Read the model definition and answer for the solid it produces. Units are mm, in the model's axes. Give positions to 0.01 mm unless a question says otherwise; leave off trailing zeros. Loops run counter-clockwise (first coordinate to the right, second up) from the corner with the lowest first, then second, coordinate; pieces in that order, holes last. Notation, with made-up numbers: (43.5, -13) - (54.5, -13) arc R34 cw to (54.5, 21) - close; hole circle Ø6 at (73, 47). An arc over 180 degrees is marked (long way). Write item = value, one per line.
```python
from build123d import *

# Parameters (mm, degrees)
EXTRUDE_1_DEPTH = 55
FILLET_1_R      = 5


with BuildPart() as part:
    # ｽｹｯﾁ1 → ﾎﾞｽ - 押し出し1 (new body)
    with BuildSketch(Plane.XY):
        with BuildLine():
            Line((61.949000384, 214.222597667), (62.393477517, 215.75962079))
            ThreePointArc((62.393477517, 215.75962079), (0, 224.6), (-62.393477517, 215.75962079))
            Line((-62.393477517, 215.75962079), (-61.949000384, 214.222597667))
            ThreePointArc((-61.949000384, 214.222597667), (0, 223), (61.949000384, 214.222597667))
        make_face()
    extrude(amount=EXTRUDE_1_DEPTH)

    # ﾌｨﾚｯﾄ1
    fillet_1_edges = [part.edges().sort_by_distance(p)[0] for p in [
        (-62.171238951, 214.991109229, 55),
        (-62.171238951, 214.991109229, 0),
        (62.171238951, 214.991109229, 0),
        (62.171238951, 214.991109229, 55),
    ]]
    fillet(fillet_1_edges, radius=FILLET_1_R)

    # ｽｹｯﾁ2 → ｶｯﾄ - 回転1 (revolve, cut)
    with BuildSketch(Plane.XY.offset(27.5), mode=Mode.PRIVATE) as cut_revolve_1_sk:
        Polygon((51.528577079, 205.436232793), (57.367509326, 228.715126027), (54.457647672, 229.444992558), (48.618715425, 206.166099324), align=None)
    revolve(cut_revolve_1_sk.sketch.rotate(Axis((51.528577079, 205.436232793, 27.5), (0.24328884362241038, 0.9699538847640492, 0)), 180), axis=Axis((51.528577079, 205.436232793, 27.5), (0.24328884362241038, 0.9699538847640492, 0)), mode=Mode.SUBTRACT)

    # ｽｹｯﾁ3 → ｶｯﾄ - 回転2 (revolve, cut)
    with BuildSketch(Plane.XY.offset(27.5), mode=Mode.PRIVATE) as cut_revolve_2_sk:
        Polygon((-51.528577079, 205.436232793), (-57.367509326, 228.715126027), (-60.27737098, 227.985259496), (-54.438438734, 204.706366262), align=None)
    revolve(cut_revolve_2_sk.sketch.rotate(Axis((-51.528577079, 205.436232793, 27.5), (-0.24328884362241038, 0.9699538847640492, 0)), 180), axis=Axis((-51.528577079, 205.436232793, 27.5), (-0.24328884362241038, 0.9699538847640492, 0)), mode=Mode.SUBTRACT)


solid = part.part
```
1) The mould has two halves that part along Z. Classify faces 1 (the face through (52.3, 217.59, 25.47)), 2 (the face through (-0.3, 223.4, 55)), 3 (the face through (-0.3, 223.4, 0)): pulls with the +Z half, pulls with the -Z half, needs draft (parallel to the pull), parting line crosses it, or undercut.
Output:
face_1 = undercut
face_2 = pulls with the +Z half
face_3 = pulls with the -Z half
2) A cutting plane is placed at B-B on z = 20. Determine the outline of the cut face in (x, y).
Output:
outline = (-62.39, 215.76) - (-61.95, 214.22) arc R223 cw to (61.95, 214.22) - (62.39, 215.76) arc R224.6 ccw to start
3) This flat-tipped pin is pushed along its axis until it touches: P1, Ø4, axis at x = -42.5, y = 216.5, coming from the +Z side. Where does it stop, or does it pass through?
Output:
P1 = through
4) Find the intervals of material crossed by probe 1 along Z at (x, y) = (52.5, 217) (3 decimals); probe 2 along Y at (x, z) = (38.5, 29.5); probe 3 along Y at (x, z) = (28, 18), in increasing order.
Output:
probe_1 = 0 to 25.155, 29.845 to 55
probe_2 = 219.65 to 221.28
probe_3 = 221.24 to 222.85
5) A cutting plane is placed at A-A on y = 219.75. Determine the outline of the cut face in (x, z).
Output:
outline = (-46.42, 0) - (-37.93, 0) - (-37.93, 55) - (-46.42, 55) - close; (37.93, 0) - (46.42, 0) - (46.42, 55) - (37.93, 55) - close
6) A cutting plane is placed at C-C on x = 48. Determine the outline of the cut face in (y, z).
Output:
outline = (217.77, 0) - (219.41, 0) - (219.41, 55) - (217.77, 55) - close
